from build123d import *

# Parameters (mm, degrees)
F0_R     = 55
F0_R_2   = 53
F1_DEPTH = 15
F2_R     = 55
F2_R_2   = 53
F3_DEPTH = 2
F4_W     = 10
F4_H     = 15
F5_ANGLE = 180
F7_DEPTH = 15


with BuildPart() as f1:
    # F0 (on Top) → F1 (new body)
    with BuildSketch(Plane.XY):
        Circle(F0_R)
        Circle(F0_R_2, mode=Mode.SUBTRACT)
        Circle(F0_R_2)
    extrude(amount=F1_DEPTH)

    # F2 (on Top) → F3 (join)
    with BuildSketch(Plane.XY):
        Circle(F2_R)
        Circle(F2_R_2, mode=Mode.SUBTRACT)
    extrude(amount=-F3_DEPTH)

    # F4 (on face) → F5 (revolve)
    with BuildSketch(Plane.XY.offset(15)):
        with Locations((-20, 7.5)):
            Rectangle(F4_W, F4_H)
        with Locations((20, 7.5)):
            Rectangle(F4_W, F4_H)
    revolve(axis=Axis((3.316946, 0, 15), (1, 0, 0)), revolution_arc=F5_ANGLE)

    # F6 (on Top) → F7 (join)
    with BuildSketch(Plane.XY):
        Polygon((-70, 6.5), (-53.270391, 6.5), (-52.225381, 9.5), (-73, 9.5), (-73, 0), (-73, -9.5), (-52.225381, -9.5), (-53.270391, -6.5), (-70, -6.5), (-70, 0), align=None)
        Polygon((73, 9.5), (52.225381, 9.5), (53.270391, 6.5), (70, 6.5), (70, 0), (70, -6.5), (53.270391, -6.5), (52.225381, -9.5), (73, -9.5), (73, 0), align=None)
    extrude(amount=F7_DEPTH)


solid = f1.part
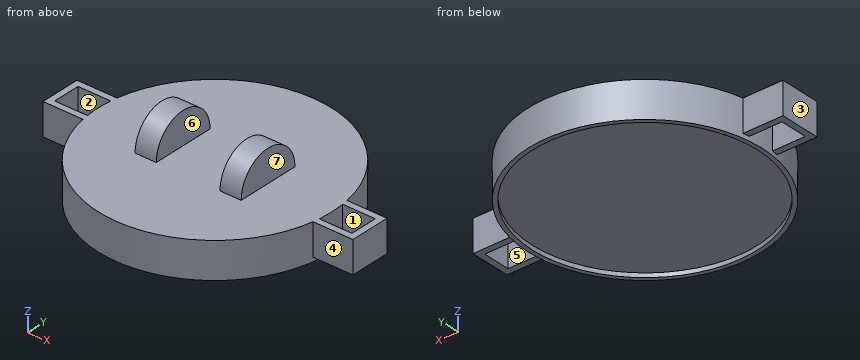
Verification items for the finished model (mm, model axes). Face numbers are marked on the shaded views. A direction names the side the tool comes from. Coordinates: 2 decimals unless noted, no trailing zeros. Write each loop counter-clockwise with the first axis right and the second up, starting at its lowest first coordinate (ties: lowest second). Pieces come first, ordered by that corner, then holes. Notation, with made-up numbers: M -21,52 L -12,52 A18 cw -12,74 Z; hole C 23.25,43 d2. An arc over 180 degrees is marked long. Use CSV: the item, a comma, the result in double quotes.
Q1. Thickness scan on line 1 along Y through (x, z) = (0, -1.3); line 2 along X through (y, z) = (-10, 19); line 3 along X through (y, z) = (4, 5). Record the ranges inside material, lowest first. Write a range as [from, to].
Computed values:
line 1,"[-55, -53], [53, 55]"
line 2,"[-25, -15], [15, 25]"
line 3,"[-73, -70], [-54.85, 54.85], [70, 73]"
Q2. Section check C-C, the plane y = 0. Enter the section's corners in (x, z), and give its area (3 significant figures).
Computed values:
outline,"M -73,0 L -70,0 L -70,15 L -73,15 Z; M -55,-2 L -53,-2 L -53,0 L 53,0 L 53,-2 L 55,-2 L 55,15 L 25,15 L 25,30 L 15,30 L 15,15 L -15,15 L -15,30 L -25,30 L -25,15 L -55,15 Z; M 70,0 L 73,0 L 73,15 L 70,15 Z"
area,"2,050 mm²"
Q3. Mould release check, pull along Y, two halves, no side actions. Record for the marked faces 1, 2, 3 and 4: pulls with the +Y half, pulls with the -Y half, needs draft (parallel to the pull), parting line crosses it, or undercut.
Computed values:
face 1,"undercut"
face 2,"undercut"
face 3,"needs draft"
face 4,"pulls with the -Y half"
Q4. Section check B-B, the plane z = 1.5. Enter the section's corners in (x, y), and give its area (3 significant figures).
Computed values:
outline,"M -73,-9.5 L -54.17,-9.5 A55 ccw 54.17,-9.5 L 73,-9.5 L 73,9.5 L 54.17,9.5 A55 ccw -54.17,9.5 L -73,9.5 Z; hole M -70,-6.5 L -54.61,-6.5 A55 cw -54.61,6.5 L -70,6.5 Z; hole M 54.61,-6.5 L 70,-6.5 L 70,6.5 L 54.61,6.5 A55 cw Z"
area,"9,800 mm²"
Q5. Section check A-A, the plane x = -57.5. Enter the section's corners in (y, z).
Computed values:
outline,"M -9.5,0 L -6.5,0 L -6.5,15 L -9.5,15 Z; M 6.5,0 L 9.5,0 L 9.5,15 L 6.5,15 Z"
Q6. Section check D-D, the plane x = 0. Enter the section's corners in (y, z).
Computed values:
outline,"M -55,-2 L -53,-2 L -53,0 L 53,0 L 53,-2 L 55,-2 L 55,15 L -55,15 Z"
Q7. Set-up check for the marked faces 5, 6 and 7: record each of +Z, -Z, +X, -X, +Y, -Y from which the full face is reachable in a straight line by a thin tool's end or side.
Computed values:
face 5,"+Z, -Z"
face 6,"+Z, +Y, -Y"
face 7,"+Z, +X, +Y, -Y"
Q8. Go/stop test with flat-tipped pins: P1, Ø12, axis at y = -4, z = 23, coming from the +X side; P2, Ø12, axis at x = -38.5, z = 8.5, coming from the +Y side; P3, Ø12, axis at x = -32, z = 14.5, coming from the +Y side; P4, Ø16.5, axis at y = 5, z = 20.5, coming from the +X side. Record where each tip stops, or that it passes through.
Computed values:
P1,"x = 25"
P2,"y = 44.37"
P3,"y = 48.47"
P4,"x = 73"
